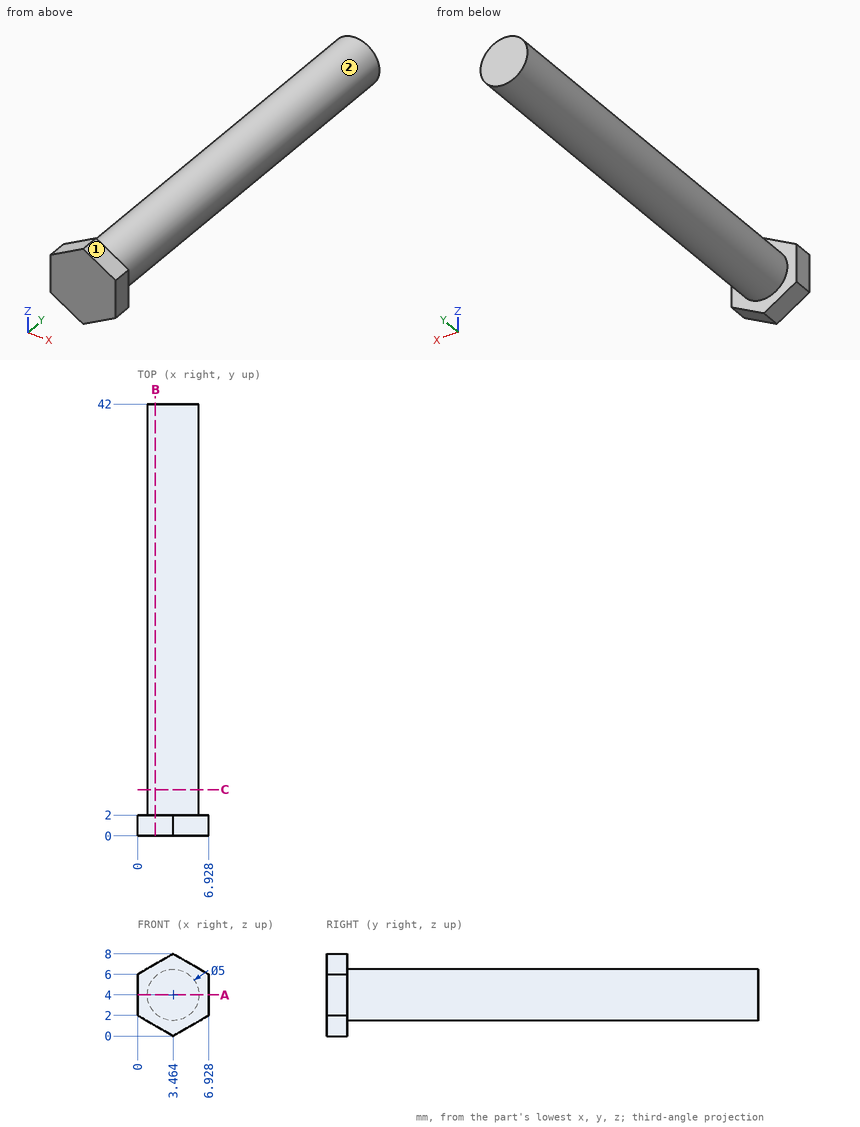
Here's the drawing with two shaded views (mm, measured from the low corner). I have some questions. A direction names the side the tool comes from. Give positions to 0.01 mm unless a question says otherwise; leave off trailing zeros. Loops run counter-clockwise (first coordinate to the right, second up) from the corner with the lowest first, then second, coordinate; pieces in that order, holes last. Notation, with made-up numbers: M -17.5,61 L 3.5,61 A20 ccw 3.5,82 Z; hole C 3.5,22 d3. An arc over 180 degrees is marked long. Use one line per item in the form item = value. Start each with the question number.
Q1. Which directions (+Z, -Z, +X, -X, +Y, -Y) give clear straight access to the entire face, cutting with the end or side of a thin tool? Please do the marked faces 1 and 2.
Q2. If we section it at A-A (z = 4): Write out the boundary of the cut face in (x, y).
Q3. If we section it at C-C (y = 4.5): Write out the boundary of the cut face in (x, z), then the cut area to 3 significant figures.
Q4. I need wall thicknesses on line 1 along Y through (x, z) = (5.25, 2); line 2 along Z through (x, y) = (3.5, 37.5); line 3 along Z through (x, y) = (4.75, 35.5). Which ranges of each line are inside material? Lowest first, please.
Q5. If we section it at B-B (x = 1.75): Write out the boundary of the cut face in (y, z).
Q6. Will these pins go through, and if not, where does the flat tip stop? pin 1 Ø4 at (y, z) = (27.5, 2.5) entering from -X; pin 2 Ø1.5 at (x, y) = (4, 25.5) entering from +Z; pin 3 Ø1.5 at (x, y) = (6, 29) entering from +Z.
Taken from the geometry:
q1.face_1 = +Z, +X, +Y, -Y
q1.face_2 = +Y
q2.outline = M 0,0 L 6.93,0 L 6.93,2 L 5.96,2 L 5.96,42 L 0.96,42 L 0.96,2 L 0,2 Z
q3.outline = C 3.46,4 d5
q3.area = 19.6 mm^2
q4.line_1 = 0 to 2
q4.line_2 = 1.5 to 6.5
q4.line_3 = 1.86 to 6.14
q5.outline = M 0,0.99 L 2,0.99 L 2,2.18 L 42,2.18 L 42,5.82 L 2,5.82 L 2,7.01 L 0,7.01 Z
q6.pin_1 = 0.96
q6.pin_2 = 6.5
q6.pin_3 = 5.75
